Design review of the part built by this model. Coordinates are the model's own, in mm. A direction names the side the tool comes from. Coordinates: 2 decimals unless noted, no trailing zeros. Loops run counter-clockwise (first coordinate to the right, second up) from the corner with the lowest first, then second, coordinate; pieces in that order, holes last. Notation, with made-up numbers: M 16.25,19 L 27.25,19 A31 cw 27.25,43 Z; hole C 83.25,34.5 d11. An arc over 180 degrees is marked long. Answer as a JSON object with one key per item and string values. Group by question number.
1. Draft analysis for pull direction X (two halves, no side actions). For faces 1 (the flat face through (2, 100, 1496)), 2 (the cylindrical face through (106.56, 50.7, 1496.21)), 3 (the cylindrical face through (-35.6, 25.02, 1538.67)), state which applies: +X half, -X half, draft (parallel to the pull), parting line (faces both ways), or undercut.
2. Consider section D-D (x = -35). State the section outline as (y, z) points, then the cut area to 3 significant figures.
3. Consider section B-B (y = 68). State the section outline as (x, z) points, then the cut area to 3 significant figures.
4. Consider section A-A (z = 1432). State the section outline as (x, y) points, then the cut area to 3 significant figures.
5. Machinability: for faces 4 (the flat face through (12.5, 51, 1425)), 5 (the cylindrical face through (-108.35, 50.7, 1521.3)), 6 (the flat face through (136.14, 49.3, 1556.11)), 7 (the flat face through (-126.437, 49.3, 1445.18)), 8 (the cylindrical face through (35.6, 25.02, 1538.67)), which of the approach directions +Z, -Z, +X, -X, +Y, -Y give a long, thin tool a straight path to every point of the face, cutting with its end or side? Answer none if there is none.
6. Insertion check: pin 1 (1 mm diameter, centred on y = 76, z = 1493.5, fed in from +X); pin 2 (25 mm diameter, centred on y = 39, z = 1432.5, fed in from +X); pin 3 (12 mm diameter, centred on y = 22.5, z = 1575, fed in from +X); pin 4 (24.5 mm diameter, centred on x = -35, z = 1525, fed in from +Y). Each pin has a flat end and moves straight along its axis. Give the tip position at first contact, or say it passes through.
7. To check wall thickness, follow probe 1 along X at (y, z) = (68, 1528.5); probe 2 along X at (y, z) = (11, 1525); probe 3 along Z at (x, y) = (-44.5, 52). State the ranges of each line that lie inside material, in increasing order.
8. Consider section C-C (x = 102). State the section outline as (y, z) points, then the cut area to 3 significant figures.
from build123d import *

# Parameters (mm, degrees)
EXTRUDE_1_DEPTH     = 100
CUT_EXTRUDE_2_DEPTH = 1610.175588972
CUT_EXTRUDE_3_DEPTH = 1610.175588972


with BuildPart() as part:
    # 草图3 → 凸台-拉伸1 (new body)
    with BuildSketch(Plane(origin=(0, 0, 0), x_dir=(1, 0, 0), z_dir=(0, 1, 0))):
        with BuildLine():
            Line((-139.449188396, -1593.911516947), (-122.018039847, -1394.672577328))
            ThreePointArc((-122.018039847, -1394.672577328), (0, -1400), (122.018039847, -1394.672577328))
            Line((122.018039847, -1394.672577328), (139.449188396, -1593.911516947))
            ThreePointArc((139.449188396, -1593.911516947), (0, -1600), (-139.449188396, -1593.911516947))
        make_face()
    extrude(amount=EXTRUDE_1_DEPTH)

    # 草图6 → 切除-拉伸2 (cut, through all)
    with BuildSketch(Plane(origin=(0, 100, 0), x_dir=(1, 0, 0), z_dir=(0, 1, 0))):
        Polygon((-12.5, -1399.944195316), (12.5, -1399.944195316), (12.5, -1449.944195316), (0, -1449.944195316), (-12.5, -1449.944195316), align=None)
    extrude(amount=-CUT_EXTRUDE_2_DEPTH, mode=Mode.SUBTRACT)

    # 草图8 → 切除-旋转1 (revolve, cut)
    with BuildSketch(Plane(origin=(-35, 0, 0), x_dir=(0, 0, -1), z_dir=(1, 0, 0)), mode=Mode.PRIVATE) as cut_revolve_1_sk:
        Polygon((-1525, 100), (-1530, 100), (-1538.682408883, 50.759612349), (-1538.682408883, 0), (-1525, 0), align=None)
    cut_revolve_1 = revolve(cut_revolve_1_sk.sketch.rotate(Axis((-35, 0, 1525), (0, 1, 0)), 180), axis=Axis((-35, 0, 1525), (0, 1, 0)), mode=Mode.SUBTRACT)

    # 镜向1: 切除-旋转1 across plane
    add(cut_revolve_1.mirror(Plane.ZY), mode=Mode.SUBTRACT)

    # 草图9 → 切除-拉伸3 (cut, through all)
    with BuildSketch(Plane(origin=(0, 100, 0), x_dir=(1, 0, 0), z_dir=(0, 1, 0))):
        with BuildLine():
            Line((81.67512146, -1497.774740919), (83.044783982, -1522.891886672))
            ThreePointArc((83.044783982, -1522.891886672), (107.999891135, -1521.325789617), (132.925969989, -1519.350789364))
            Line((132.925969989, -1519.350789364), (130.733614121, -1494.292047138))
            ThreePointArc((130.733614121, -1494.292047138), (106.218642558, -1496.234473595), (81.67512146, -1497.774740919))
        make_face()
        with BuildLine():
            Line((-83.044783982, -1522.891886672), (-81.67512146, -1497.774740919))
            ThreePointArc((-81.67512146, -1497.774740919), (-106.218642558, -1496.234473595), (-130.733614121, -1494.292047138))
            Line((-130.733614121, -1494.292047138), (-132.925969989, -1519.350789364))
            ThreePointArc((-132.925969989, -1519.350789364), (-107.999891135, -1521.325789617), (-83.044783982, -1522.891886672))
        make_face()
    extrude(amount=-CUT_EXTRUDE_3_DEPTH, mode=Mode.SUBTRACT)


solid = part.part
Findings below:
{
 "1": {"face 1": "draft", "face 2": "+X half", "face 3": "undercut"},
 "2": {"outline": "M 0,1399.56 L 100,1399.56 L 100,1520 L 50.76,1511.32 L 0,1511.32 Z; M 0,1538.68 L 50.76,1538.68 L 100,1530 L 100,1599.62 L 0,1599.62 Z", "area": "17,700 mm^2"},
 "3": {"outline": "M -139.45,1593.91 L -132.93,1519.35 A1525.15 cw -83.04,1522.89 L -81.68,1497.77 A1500 ccw -130.73,1494.29 L -122.02,1394.67 A1400 cw -12.5,1399.94 L -12.5,1449.94 L 12.5,1449.94 L 12.5,1399.94 A1400 cw 122.02,1394.67 L 130.73,1494.29 A1500 ccw 81.68,1497.77 L 83.04,1522.89 A1525.15 cw 132.93,1519.35 L 139.45,1593.91 A1600 ccw Z; hole C -35,1525 d21.28; hole C 35,1525 d21.28", "area": "47,900 mm^2"},
 "4": {"outline": "M -125.28,0 L -12.5,0 L -12.5,100 L -125.28,100 Z; M 12.5,0 L 125.28,0 L 125.28,100 L 12.5,100 Z", "area": "22,600 mm^2"},
 "5": {"face 4": "-Z, +Y, -Y", "face 5": "+Y, -Y", "face 6": "-Z, +X, +Y, -Y", "face 7": "-Z, -X, +Y, -Y", "face 8": "-Y"},
 "6": {"pin 1": "stops at x = 130.71", "pin 2": "stops at x = 126.42", "pin 3": "stops at x = 138.32", "pin 4": "stops at y = 100"},
 "7": {"probe 1": "x = -133.73 to -45.05, -24.95 to 24.95, 45.05 to 133.73", "probe 2": "x = -133.42 to -48.68, -21.32 to 21.32, 48.68 to 133.42", "probe 3": "z = 1399.29 to 1515.46, 1534.54 to 1599.38"},
 "8": {"outline": "M 0,1396.28 L 100,1396.28 L 100,1496.53 L 0,1496.53 Z; M 0,1521.74 L 100,1521.74 L 100,1596.75 L 0,1596.75 Z", "area": "17,500 mm^2"}
}
